Autodesk Inventor part; units mm, degrees
ref_plane "YZ Plane" through (0, 0, 0) normal (1, 0, 0) x (0, 1, 0)
ref_plane "XZ Plane" through (0, 0, 0) normal (0, 1, 0) x (-1, 0, 0)
ref_plane "XY Plane" through (0, 0, 0) normal (0, 0, 1) x (1, 0, 0)
sketch "Sketch1" plane through (0, 0, 0) normal (0, 0, 1) x (1, 0, 0)
  line L0 (8, -8) -> (-8, -8)
  line L1 (-8, -8) -> (-8, 8)
  line L2 (-8, 8) -> (8, 8)
  line L3 (8, 8) -> (8, -8)
  line L4 (8, -8) -> (-8, 8) construction
  line L5 (-8, -8) -> (8, 8) construction
  point P0 (0, 0)
  dimension "d0" = 16
  dimension "d1" = 16
extrude "Extrusion1" add sketch "Sketch1" along normal blind 96
sketch "Sketch2" plane through (0, 0, 96) normal (0, 0, 1) x (1, 0, 0)
  line L0 (6, -6) -> (-6, -6)
  line L1 (-6, -6) -> (-6, 6)
  line L2 (-6, 6) -> (6, 6)
  line L3 (6, 6) -> (6, -6)
  line L4 (6, -6) -> (-6, 6) construction
  line L5 (-6, -6) -> (6, 6) construction
  point P0 (0, 0)
  dimension "d4" = 12
  dimension "d5" = 12
extrude "Extrusion2" cut sketch "Sketch2" against normal blind 96
sketch "Sketch9" plane through (-8, -8, 0) normal (0, -1, 0) x (1, 0, 0)
  circle A0 centre (8, 0) radius 4
  dimension "d52" = 8
hole "Hole7" at (0, -8, 0) direction (0, 1, 0) diameter 8 end through all
sketch "Sketch10" plane through (8, -8, 0) normal (1, 0, 0) x (0, 0, -1)
  circle A0 centre (0, 8) radius 4
  dimension "d60" = 8
hole "Hole8" at (8, 0, 0) direction (-1, 0, 0) diameter 8 end through all
sketch "Sketch11" plane through (-8, -8, 96) normal (0, -1, 0) x (1, 0, 0)
  circle A0 centre (8, -88) radius 1.85
  circle A1 centre (8, -72) radius 1.85
  circle A2 centre (8, -56) radius 1.85
  circle A3 centre (8, -40) radius 1.85
  circle A4 centre (8, -24) radius 1.85
  circle A5 centre (8, -8) radius 1.85
  point P0 (8, -96)
hole "Hole9" at (0, -8, 8) at (0, -8, 24) at (0, -8, 40) at (0, -8, 56) at (0, -8, 72) at (0, -8, 88) direction (0, 1, 0) diameter 3.7 end through all
sketch "Sketch12" plane through (-8, -8, 96) normal (0, -1, 0) x (1, 0, 0)
  circle A0 centre (8, -80) radius 4
  circle A1 centre (8, -64) radius 4
  circle A2 centre (8, -48) radius 4
  circle A3 centre (8, -32) radius 4
  circle A4 centre (8, -16) radius 4
  circle A5 centre (8, 0) radius 4
  point P0 (8, -96)
hole "Hole10" at (0, -8, 16) at (0, -8, 32) at (0, -8, 48) at (0, -8, 64) at (0, -8, 80) at (0, -8, 96) direction (0, 1, 0) diameter 8 end through all
sketch "Sketch13" plane through (8, -8, 96) normal (1, 0, 0) x (0, 0, -1)
  circle A0 centre (88, 8) radius 1.85
  circle A1 centre (72, 8) radius 1.85
  circle A2 centre (56, 8) radius 1.85
  circle A3 centre (40, 8) radius 1.85
  circle A4 centre (24, 8) radius 1.85
  circle A5 centre (8, 8) radius 1.85
  point P0 (96, 8)
hole "Hole11" at (8, 0, 8) at (8, 0, 24) at (8, 0, 40) at (8, 0, 56) at (8, 0, 72) at (8, 0, 88) direction (-1, 0, 0) diameter 3.7 end through all
sketch "Sketch14" plane through (8, -8, 96) normal (1, 0, 0) x (0, 0, -1)
  circle A0 centre (80, 8) radius 4
  circle A1 centre (64, 8) radius 4
  circle A2 centre (48, 8) radius 4
  circle A3 centre (32, 8) radius 4
  circle A4 centre (16, 8) radius 4
  circle A5 centre (0, 8) radius 4
  point P0 (96, 8)
hole "Hole12" at (8, 0, 16) at (8, 0, 32) at (8, 0, 48) at (8, 0, 64) at (8, 0, 80) at (8, 0, 96) direction (-1, 0, 0) diameter 8 end through all
properties part number "cube channel short"
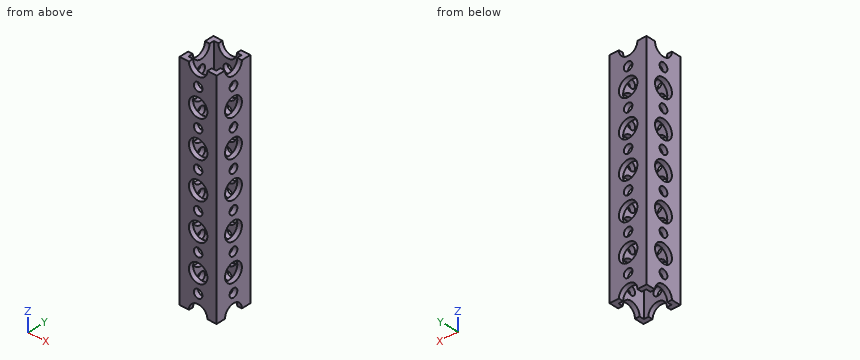
The listing builds one solid part. Answer for the finished solid, in the listing's coordinates (mm). Round coordinates to 2 decimals unless told otherwise and drop trailing zeros. Order: outer loops, then holes, each group sorted by start corner. A loop starts at its lowest first (then second) coordinate and runs counter-clockwise, first axis right, second up. Notation, with made-up numbers: (27, -37) - (74, -37) arc R30 cw to (74, -1) - close; hole circle Ø9 at (42, 48.25). An arc over 180 degrees is marked (long way). Put each result on its own line as item: value. Start each with the question number.
(1) Find section A-A (z = 24). Give the vertices of the cut face in (x, y).
(2) Find section C-C (z = 80). Give the vertices of the cut face in (x, y), plus the area to 3 significant figures.
(3) Straight lines are drawn through the part: probe 1 along Y at (x, z) = (4.25, 44); probe 2 along Y at (x, z) = (-7.45, 88). For each, find the intervals that lie inside material, in ascending order. Write a range as from..to.
(4) Find section B-B (y = 0). State how many separate pieces and enclosed holes the cut face has, plus the area to 3 significant figures.
(5) Given P1, Ø2, axis at y = 0, z = 24, coming from the +X side, flat-ended and moving along its own axis, determine where the tip first touches the part or whether it passes through.
Reply:
1. outline: (-8, -8) - (-1.85, -8) - (-1.85, -6) - (-6, -6) - (-6, -1.85) - (-8, -1.85) - close; (-8, 1.85) - (-6, 1.85) - (-6, 6) - (-1.85, 6) - (-1.85, 8) - (-8, 8) - close; (1.85, -8) - (8, -8) - (8, -1.85) - (6, -1.85) - (6, -6) - (1.85, -6) - close; (1.85, 6) - (6, 6) - (6, 1.85) - (8, 1.85) - (8, 8) - (1.85, 8) - close
2. outline: (-8, -8) - (-4, -8) - (-4, -6) - (-6, -6) - (-6, -4) - (-8, -4) - close; (-8, 4) - (-6, 4) - (-6, 6) - (-4, 6) - (-4, 8) - (-8, 8) - close; (4, -8) - (8, -8) - (8, -4) - (6, -4) - (6, -6) - (4, -6) - close; (4, 6) - (6, 6) - (6, 4) - (8, 4) - (8, 8) - (4, 8) - close
2. area: 48.0 mm^2
3. probe 1: -8..-6, 6..8
3. probe 2: -8..-1.85, 1.85..8
4. separate pieces: 24
4. enclosed holes: 0
4. area: 103 mm^2
5. P1: through
